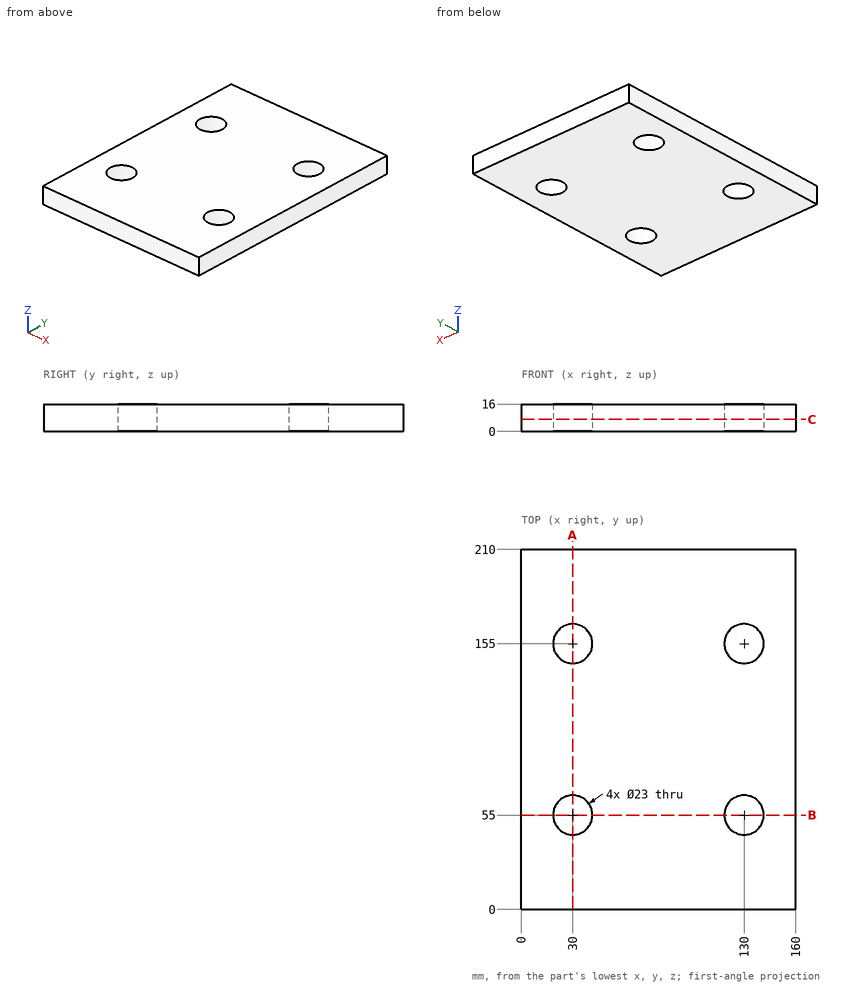
Verification items for this drawing (mm, ordinates from the low corner). Coordinates: 2 decimals unless noted, no trailing zeros. Order: outer loops, then holes, each group sorted by start corner. A loop starts at its lowest first (then second) coordinate and runs counter-clockwise, first axis right, second up.
Q1. Thickness scan on probe 1 along Y at (x, z) = (130, 4); probe 2 along Y at (x, z) = (120.5, 2.75); probe 3 along X at (y, z) = (160.5, 15). Record the ranges inside material, lowest first.
Reply:
probe 1: y = 0 to 43.5, 66.5 to 143.5, 166.5 to 210
probe 2: y = 0 to 48.52, 61.48 to 148.52, 161.48 to 210
probe 3: x = 0 to 19.9, 40.1 to 119.9, 140.1 to 160
Q2. Sectioned sample at A-A on x = 30. Record the cut outline in (y, z).
Reply:
outline: (0, 0) - (43.5, 0) - (43.5, 16) - (0, 16) - close; (66.5, 0) - (143.5, 0) - (143.5, 16) - (66.5, 16) - close; (166.5, 0) - (210, 0) - (210, 16) - (166.5, 16) - close
Q3. Sectioned sample at B-B on y = 55. Record the cut outline in (x, z), and give its area (3 significant figures).
Reply:
outline: (0, 0) - (18.5, 0) - (18.5, 16) - (0, 16) - close; (41.5, 0) - (118.5, 0) - (118.5, 16) - (41.5, 16) - close; (141.5, 0) - (160, 0) - (160, 16) - (141.5, 16) - close
area: 1,820 mm2
Q4. Sectioned sample at C-C on z = 7. Record the cut outline in (x, y), and give its area (3 significant figures).
Reply:
outline: (0, 0) - (160, 0) - (160, 210) - (0, 210) - close; hole circle Ø23 at (30, 55); hole circle Ø23 at (30, 155); hole circle Ø23 at (130, 55); hole circle Ø23 at (130, 155)
area: 31,900 mm2
Q5. Depth check by flat-ended pin: pin 1 Ø12 at (x, y) = (133, 155) entering from +Z. Enter the tip coordinate at first touch or a pass-through.
Reply:
pin 1: passes through
